Build history of the part. All positions in model axes, mm. Face numbers are marked on the shaded views. A direction names the side the tool comes from. Give positions to 0.01 mm unless a question says otherwise; leave off trailing zeros. Write each loop counter-clockwise with the first axis right and the second up, starting at its lowest first coordinate (ties: lowest second). Pieces come first, ordered by that corner, then holes. Notation, with made-up numbers: (68.25, 59.5) -> (77.25, 59.5) arc R21 cw to (77.25, 76.5) -> close; hole circle Ø3 at (-22.75, 42). An arc over 180 degrees is marked (long way). One line per question, with ' | ' between items. Start each with the question number.
(1) Tool access for the marked faces 4, 5 and 6: list every direction of +Z, -Z, +X, -X, +Y, -Y with a clear straight run to the whole face (end or side of a thin tool).
(2) Band-saw the part on B-B, the plane z = 12.6. Give the cut face in (x, y).
(3) Band-saw the part on A-A, the plane x = 24.1. Give the cut face in (y, z).
(4) Pull direction X, two halves, no side cores. Call the marked faces 1, 2 and 3: released by +X, released by -X, zero draft, split by the parting line, or undercut.
(5) Drill centre lines: probe 1 along X at (y, z) = (0, 24.35); probe 2 along Y at (x, z) = (-2.5, 7.75); probe 3 along Z at (x, y) = (28.5, -1.5). Where is each one in solid material? Low to high. Write a range as from..to.
(6) Band-saw the part on C-C, the plane y = -5.5. Give the cut face in (x, z).
(7) Band-saw the part on D-D, the plane x = 0. Give the cut face in (y, z), and give its area (3 significant figures).
from build123d import *

# Parameters (mm, degrees)
SKETCH1_W               = 25.2
SKETCH1_H               = 25.2
SKETCH1_W_2             = 19.2
SKETCH1_H_2             = 19.2
BOSS_EXTRUDE1_DEPTH     = 25.2
SKETCH3_W               = 25.2
SKETCH3_H               = 25.2
SKETCH3_W_2             = 19.2
SKETCH3_H_2             = 19.2
BOSS_EXTRUDE2_DEPTH     = 23
CUT_EXTRUDE1_DEPTH      = 49.941189197
CUT_EXTRUDE1_DEPTH_BACK = 49.941189197
SKETCH4_R               = 1.5875
CUT_EXTRUDE2_DEPTH      = 44.805935671
CUT_EXTRUDE2_DEPTH_BACK = 44.805935671
SKETCH5_R               = 1.5875


with BuildPart() as part:
    # Sketch1 → Boss-Extrude1 (new body)
    with BuildSketch(Plane.XY):
        Rectangle(SKETCH1_W, SKETCH1_H)
        Rectangle(SKETCH1_W_2, SKETCH1_H_2, mode=Mode.SUBTRACT)
    extrude(amount=BOSS_EXTRUDE1_DEPTH)

    # Sketch3 → Boss-Extrude2 (add)
    with BuildSketch(Plane(origin=(12.6, 0, 0), x_dir=(0, 0, -1), z_dir=(1, 0, 0))):
        with Locations((-12.6, 0)):
            Rectangle(SKETCH3_W, SKETCH3_H)
        with Locations((-12.6, 0)):
            Rectangle(SKETCH3_W_2, SKETCH3_H_2, mode=Mode.SUBTRACT)
    extrude(amount=BOSS_EXTRUDE2_DEPTH)

    # Sketch4 → Cut-Extrude1 (cut, two sides: drawn at the far end of the back side and taken through both)
    with BuildSketch(Plane(origin=(0, -9.6, 0), x_dir=(1, 0, 0), z_dir=(0, 1, 0)).offset(-CUT_EXTRUDE1_DEPTH_BACK)):
        with Locations(Location((0, -12.6, 0), (0, 0, 270))):
            Circle(SKETCH4_R)
    extrude(amount=CUT_EXTRUDE1_DEPTH + CUT_EXTRUDE1_DEPTH_BACK, mode=Mode.SUBTRACT)

    # Sketch5 → Cut-Extrude2 (cut, two sides: drawn at the far end of the back side and taken through both)
    with BuildSketch(Plane.XY.offset(3).offset(-CUT_EXTRUDE2_DEPTH_BACK)):
        with Locations(Location((24.1, 0, 0), (0, 0, 270))):
            Circle(SKETCH5_R)
    extrude(amount=CUT_EXTRUDE2_DEPTH + CUT_EXTRUDE2_DEPTH_BACK, mode=Mode.SUBTRACT)


solid = part.part
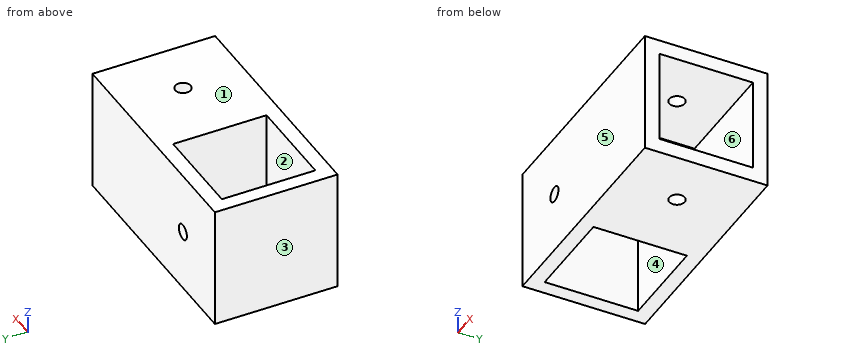
Results:
1) face 4: +Z, -Z | face 5: +Z, -Z, +X, -X, -Y | face 6: +X
2) outline: (-12.6, -12.6) -> (-1.59, -12.6) -> (-1.59, -9.6) -> (-9.6, -9.6) -> (-9.6, 9.6) -> (-1.59, 9.6) -> (-1.59, 12.6) -> (-12.6, 12.6) -> close; (1.59, -12.6) -> (35.6, -12.6) -> (35.6, -9.6) -> (12.6, -9.6) -> (12.6, 9.6) -> (35.6, 9.6) -> (35.6, 12.6) -> (1.59, 12.6) -> (1.59, 9.6) -> (9.6, 9.6) -> (9.6, -9.6) -> (1.59, -9.6) -> close
3) outline: (-12.6, 0) -> (-1.59, 0) -> (-1.59, 3) -> (-9.6, 3) -> (-9.6, 22.2) -> (-1.59, 22.2) -> (-1.59, 25.2) -> (-12.6, 25.2) -> close; (1.59, 0) -> (12.6, 0) -> (12.6, 25.2) -> (1.59, 25.2) -> (1.59, 22.2) -> (9.6, 22.2) -> (9.6, 3) -> (1.59, 3) -> close
4) face 1: zero draft | face 2: undercut | face 3: released by -X
5) probe 1: x = -12.6..-9.6, 9.6..22.51, 25.69..35.6 | probe 2: y = -12.6..-9.6, 9.6..12.6 | probe 3: z = 0..3, 22.2..25.2
6) outline: (-12.6, 0) -> (-9.6, 0) -> (-9.6, 25.2) -> (-12.6, 25.2) -> close; (9.6, 0) -> (35.6, 0) -> (35.6, 3) -> (12.6, 3) -> (12.6, 22.2) -> (35.6, 22.2) -> (35.6, 25.2) -> (9.6, 25.2) -> close
7) outline: (-12.6, 0) -> (-9.6, 0) -> (-9.6, 11.01) -> (-12.6, 11.01) -> close; (-12.6, 14.19) -> (-9.6, 14.19) -> (-9.6, 25.2) -> (-12.6, 25.2) -> close; (9.6, 0) -> (12.6, 0) -> (12.6, 11.01) -> (9.6, 11.01) -> close; (9.6, 14.19) -> (12.6, 14.19) -> (12.6, 25.2) -> (9.6, 25.2) -> close | area: 132 mm²
